Build history of the part. All positions in model axes, mm. Face numbers are marked on the shaded views. A direction names the side the tool comes from. Round coordinates to 2 decimals unless told otherwise and drop trailing zeros. Write each loop counter-clockwise with the first axis right and the second up, starting at its lowest first coordinate (ties: lowest second). Pieces come first, ordered by that corner, then holes. Notation, with made-up numbers: (58.25, -34) -> (77.25, -34) arc R8 cw to (77.25, -29) -> close; hole circle Ø8 at (32, 34.25). An arc over 180 degrees is marked (long way). Answer as CSV lines item,"result".
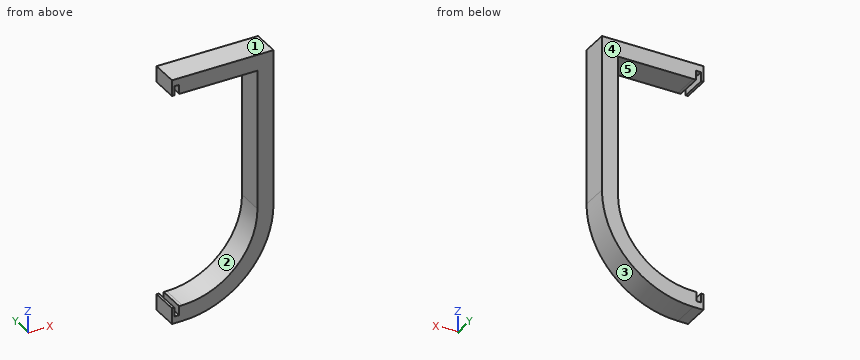
from build123d import *

# Parameters (mm, degrees)
F1_DEPTH = 25.4


with BuildPart() as f1:
    # F0 (on Front) → F1 (new body)
    with BuildSketch(Plane.XZ):
        with BuildLine():
            Line((0, -70.6374), (0, -85.678593))
            ThreePointArc((0, -85.678593), (60.583914, -60.583914), (85.678593, 0))
            Line((85.678593, 0), (70.6374, 0))
            ThreePointArc((70.6374, 0), (49.948185, -49.948185), (0, -70.6374))
        make_face()
        Polygon((70.6374, 0), (85.678593, 0), (85.678593, 131.826), (85.678593, 146.863619), (70.6374, 146.863619), (0, 146.863619), (0, 131.826819), (0, 131.826), (70.6374, 131.826), align=None)
        Polygon((-2.709501, 131.826819), (0, 131.826819), (0, 146.863619), (-9.497362, 146.863619), (-9.497362, 131.826819), (-7.281501, 131.826819), (-7.281501, 140.462819), (-2.709501, 140.462819), align=None)
        Polygon((-9.529586, -85.678593), (0, -85.678593), (0, -70.6374), (-2.745675, -70.6374), (-2.745675, -79.2734), (-7.317675, -79.2734), (-7.317675, -70.6374), (-9.529586, -70.6374), align=None)
    extrude(amount=F1_DEPTH)


solid = f1.part
1. Probe line 1 along Z through (x, y) = (-1, -22.25); line 2 along X through (y, z) = (-5.25, 121.5); line 3 along Z through (x, y) = (43, -8.5). List the from-to ranges inside material, lowest first.
Results found:
line 1,"z = -85.68 to -70.64, 131.83 to 146.86"
line 2,"x = 70.64 to 85.68"
line 3,"z = -74.11 to -56.04, 131.83 to 146.86"
2. Mould opens along Z. For the marked faces 1, 2 and 3 say: +Z half, -Z half, draft (parallel to the pull), parting line (faces both ways), or undercut.
Results found:
face 1,"+Z half"
face 2,"undercut"
face 3,"-Z half"
3. Which spindle directions (+Z, -Z, +X, -X, +Y, -Y) get a long thin tool onto all of the face, cutting with end or side? Do the marked faces 4 and 5. Say none if no direction does.
Results found:
face 4,"+Z, -Z, +X, -X, +Y"
face 5,"-X, +Y, -Y"
4. Cut at C-C, the plane z = 22.5. Write the cut outline in (x, y), then the cut area to 3 significant figures.
Results found:
outline,"(70.64, -25.4) -> (85.68, -25.4) -> (85.68, 0) -> (70.64, 0) -> close"
area,"382 mm2"
5. Cut at D-D, the plane x = 17.5. Write the cut outline in (y, z), then the cut area to 3 significant figures.
Results found:
outline,"(-25.4, -83.87) -> (0, -83.87) -> (0, -68.44) -> (-25.4, -68.44) -> close; (-25.4, 131.83) -> (0, 131.83) -> (0, 146.86) -> (-25.4, 146.86) -> close"
area,"774 mm2"
6. Cut at A-A, the plane x = 46. Write the cut outline in (y, z), then the cut area to 3 significant figures.
Results found:
outline,"(-25.4, -72.28) -> (0, -72.28) -> (0, -53.61) -> (-25.4, -53.61) -> close; (-25.4, 131.83) -> (0, 131.83) -> (0, 146.86) -> (-25.4, 146.86) -> close"
area,"856 mm2"
7. Drop flat-ended pins along their axis: pin 1 Ø8 at (x, y) = (75, -19) entering from -Z; pin 2 Ø12 at (y, z) = (-14, 143) entering from -X; pin 3 Ø5 at (y, z) = (-18.5, 22) entering from -X. Give the stop position or say it passes through.
Results found:
pin 1,"stops at z = -47.96"
pin 2,"stops at x = -9.5"
pin 3,"stops at x = 70.64"
